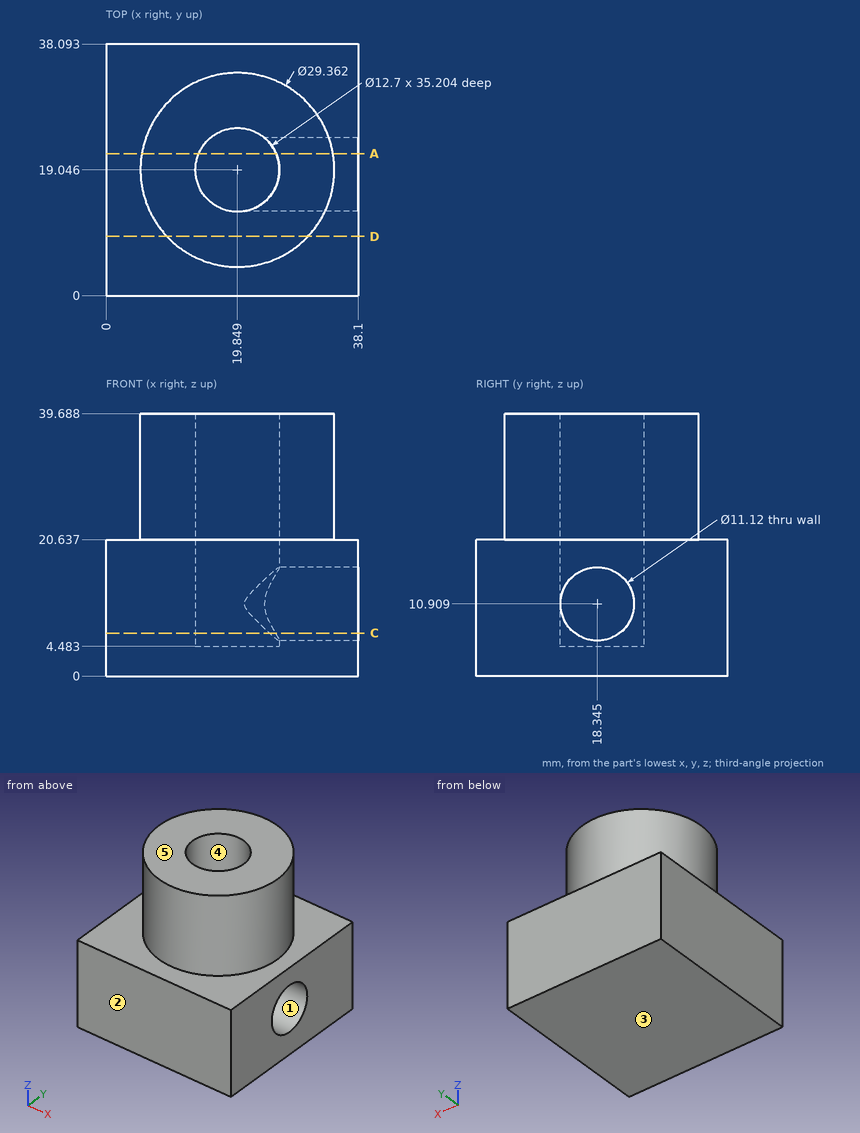
Here's the drawing with two shaded views (mm, measured from the low corner). I have some questions. A direction names the side the tool comes from. Coordinates: 2 decimals unless noted, no trailing zeros. Order: outer loops, then holes, each group sorted by start corner. A loop starts at its lowest first (then second) coordinate and runs counter-clockwise, first axis right, second up. Notation, with made-up numbers: M -11.75,43 L 4.25,43 A21 ccw 4.25,78 Z; hole C 21.25,-12.75 d5. An arc over 180 degrees is marked long. Answer as CSV lines item,"result".
Item 1: We'd pull the mould along Z, two halves only. Please class the marked faces 1, 2 and 3: +Z half, -Z half, draft (parallel to the pull), parting line (faces both ways), or undercut.
Results found:
face 1,"undercut"
face 2,"draft"
face 3,"-Z half"
Item 2: Imagine slicing it at D-D on y = 9. Write out the boundary of the cut face in (x, z) (1 decimal).
Results found:
outline,"M 0,0 L 38.1,0 L 38.1,20.6 L 30.6,20.6 L 30.6,39.7 L 9.1,39.7 L 9.1,20.6 L 0,20.6 Z"
Item 3: Imagine slicing it at A-A on y = 21.5. Write out the boundary of the cut face in (x, z) (1 decimal), plus the area to 3 significant figures.
Results found:
outline,"M 0,0 L 38.1,0 L 38.1,6.3 L 25.7,6.3 L 25.7,4.5 L 14,4.5 L 14,39.7 L 5.4,39.7 L 5.4,20.6 L 0,20.6 Z; M 25.7,15.5 L 38.1,15.5 L 38.1,20.6 L 34.3,20.6 L 34.3,39.7 L 25.7,39.7 Z"
area,"812 mm2"
Item 4: Imagine slicing it at C-C on z = 6.5. Write out the boundary of the cut face in (x, y), plus the area to 3 significant figures.
Results found:
outline,"M 0,0 L 38.1,0 L 38.1,14.96 L 24.71,14.96 A6.35 cw long 25.6,21.73 L 38.1,21.73 L 38.1,38.09 L 0,38.09 Z"
area,"1,240 mm2"
Item 5: For pin 1 (3 mm diameter, centred on y = 16.5, z = 15.5, fed in from +X); pin 2 (3 mm diameter, centred on y = 16, z = 23, fed in from -X), each with a flat end and sliding along its axis, tell me the tip position at first contact or that it passes through.
Results found:
pin 1,"x = 38.1"
pin 2,"x = 5.25"
Item 6: On a 3-axis mill with a long thin cutter (end or side, diameter ignored), from which of +Z, -Z, +X, -X, +Y, -Y can I reach the whole of each face in a straight line? I mean the marked faces 4 and 5. Say none if no direction works.
Results found:
face 4,"+Z"
face 5,"+Z, +X, -X, +Y, -Y"
Item 7: If I drill on line 1 (Z direction, x = 24, y = 23); line 2 (Z direction, x = 29.5, y = 35.5); line 3 (Y direction, x = 19.5, z = 24.5) (1 decimal), over which ranges is the centre line in solid material (lowest first)?
Results found:
line 1,"0 to 4.48"
line 2,"0 to 20.64"
line 3,"4.4 to 12.7, 25.4 to 33.7"
